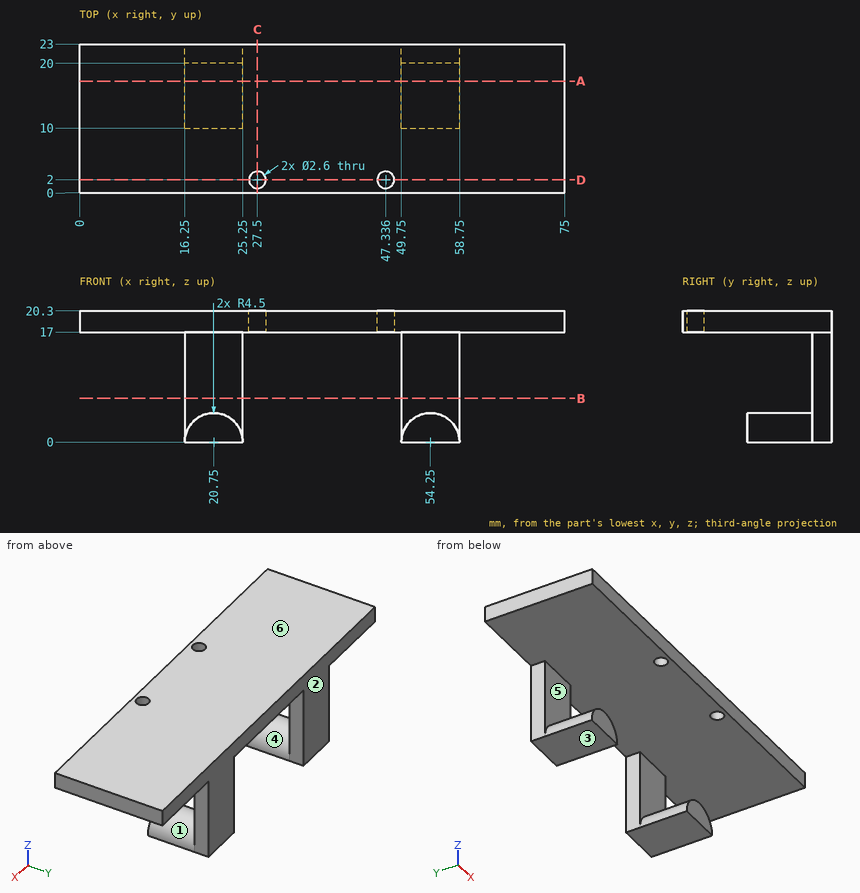
Design review of the part shown in the three views and the two pictorial views. Dimensions are in mm from the part's minimum x, y and z. A direction names the side the tool comes from. Give positions to 0.01 mm unless a question says otherwise; leave off trailing zeros. Write each loop counter-clockwise with the first axis right and the second up, starting at its lowest first coordinate (ties: lowest second). Pieces come first, ordered by that corner, then holes. Notation, with made-up numbers: (80.25, 20.25) - (132.25, 20.25) arc R23 cw to (132.25, 49.25) - close; hole circle Ø6 at (4.5, 51). An arc over 180 degrees is marked (long way). Return JSON: item names as keys, results as strings. Group by question number.
(1) Insertion check: pin 1 (1.4 mm diameter, centred on x = 56.5, z = 1, fed in from -Y); pin 2 (5 mm diameter, centred on x = 28.5, y = 4, fed in from -Z); pin 3 (2.5 mm diameter, centred on y = 22, z = 5, fed in from -X). Each pin has a flat end and moves straight along its axis. Give the tip position at first contact, or say it passes through.
(2) We need section A-A, the plane y = 17.25. Give the boundary of the cut face in (x, z), then the cut area to 3 significant figures.
(3) We need section B-B, the plane z = 6.75. Give the boundary of the cut face in (x, y).
(4) We need section D-D, the plane y = 2. Give the boundary of the cut face in (x, z), then the cut area to 3 significant figures.
(5) Mouldability with a two-part tool opening along Z and no side actions: class the marked faces 3, 4, 5 and 6 as +Z half, -Z half, draft (parallel to the pull), parting line (faces both ways), or undercut.
(6) We need section C-C, the plane x = 27.5. Give the boundary of the cut face in (y, z).
(7) Machinability: for the marked faces 1 and 2, which of the approach directions +Z, -Z, +X, -X, +Y, -Y give a long, thin tool a straight path to every point of the face, cutting with its end or side? Answer none if there is none.
(8) To check wall thickness, follow probe 1 along Y at (x, z) = (27.5, 18.8); probe 2 along X at (y, z) = (20.5, 7.5); probe 3 along Z at (x, y) = (40.5, 16.75). State the ranges of each line that lie inside material, in increasing order.
Reported:
{
 "1": {"pin 1": "stops at y = 10", "pin 2": "stops at z = 17", "pin 3": "stops at x = 16.25"},
 "2": {"outline": "(0, 17) - (75, 17) - (75, 20.3) - (0, 20.3) - close; (16.25, 0) - (25.25, 0) arc R4.5 ccw to start; (49.75, 0) - (58.75, 0) arc R4.5 ccw to start", "area": "311 mm2"},
 "3": {"outline": "(16.25, 20) - (25.25, 20) - (25.25, 23) - (16.25, 23) - close; (49.75, 20) - (58.75, 20) - (58.75, 23) - (49.75, 23) - close"},
 "4": {"outline": "(0, 17) - (26.2, 17) - (26.2, 20.3) - (0, 20.3) - close; (28.8, 17) - (46.04, 17) - (46.04, 20.3) - (28.8, 20.3) - close; (48.64, 17) - (75, 17) - (75, 20.3) - (48.64, 20.3) - close", "area": "230 mm2"},
 "5": {"face 3": "-Z half", "face 4": "undercut", "face 5": "undercut", "face 6": "+Z half"},
 "6": {"outline": "(0, 17) - (0.7, 17) - (0.7, 20.3) - (0, 20.3) - close; (3.3, 17) - (23, 17) - (23, 20.3) - (3.3, 20.3) - close"},
 "7": {"face 1": "-Y", "face 2": "+Z, -Z, +X, -X, +Y"},
 "8": {"probe 1": "y = 0 to 0.7, 3.3 to 23", "probe 2": "x = 16.25 to 25.25, 49.75 to 58.75", "probe 3": "z = 17 to 20.3"}
}
